Source: CAD feature listing. Evaluate the final solid. Frame: model axes, mm. Give positions to 0.01 mm unless a question says otherwise; leave off trailing zeros. Loops run counter-clockwise (first coordinate to the right, second up) from the corner with the lowest first, then second, coordinate; pieces in that order, holes last. Notation, with made-up numbers: M -34,11 L 10,11 A19 ccw 10,21 Z; hole C -16.5,56 d9. An arc over 180 degrees is marked long. Write item = value, one per line.
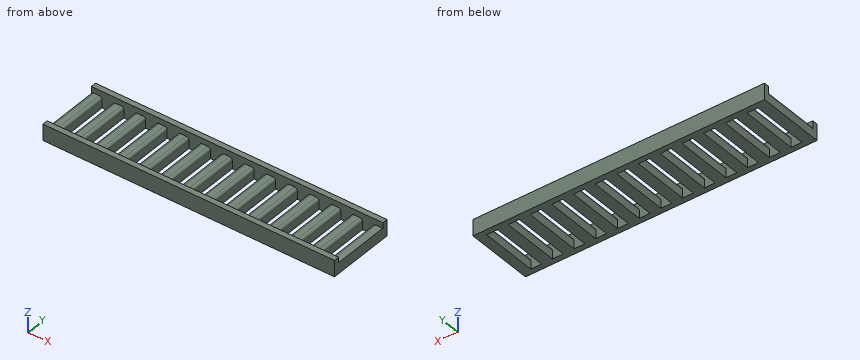
from build123d import *

# Parameters (mm, degrees)
F0_W     = 107.5
F0_H     = 25
F0_W_2   = 4
F0_H_2   = 21
F1_DEPTH = 4
F2_R     = 1
F3_W     = 107.5
F3_H     = 2
F4_DEPTH = 2
F5_R     = 1


# Not quite as in the source:
# - a feature names something its author has since deleted; it is built from what else it names


with BuildPart() as f1:
    # F0 (on Top) → F1 (new body)
    with BuildSketch(Plane.XY):
        with Locations((53.75, 12.5)):
            Rectangle(F0_W, F0_H)
        with Locations((6, 12.5)):
            Rectangle(F0_W_2, F0_H_2, mode=Mode.SUBTRACT)
        with Locations((14, 12.5)):
            Rectangle(F0_W_2, F0_H_2, mode=Mode.SUBTRACT)
        with Locations((22, 12.5)):
            Rectangle(F0_W_2, F0_H_2, mode=Mode.SUBTRACT)
        with Locations((30, 12.5)):
            Rectangle(F0_W_2, F0_H_2, mode=Mode.SUBTRACT)
        with Locations((38, 12.5)):
            Rectangle(F0_W_2, F0_H_2, mode=Mode.SUBTRACT)
        with Locations((46, 12.5)):
            Rectangle(F0_W_2, F0_H_2, mode=Mode.SUBTRACT)
        with Locations((54, 12.5)):
            Rectangle(F0_W_2, F0_H_2, mode=Mode.SUBTRACT)
        with Locations((62, 12.5)):
            Rectangle(F0_W_2, F0_H_2, mode=Mode.SUBTRACT)
        with Locations((70, 12.5)):
            Rectangle(F0_W_2, F0_H_2, mode=Mode.SUBTRACT)
        with Locations((78, 12.5)):
            Rectangle(F0_W_2, F0_H_2, mode=Mode.SUBTRACT)
        with Locations((86, 12.5)):
            Rectangle(F0_W_2, F0_H_2, mode=Mode.SUBTRACT)
        with Locations((94, 12.5)):
            Rectangle(F0_W_2, F0_H_2, mode=Mode.SUBTRACT)
        with Locations((102, 12.5)):
            Rectangle(F0_W_2, F0_H_2, mode=Mode.SUBTRACT)
    extrude(amount=F1_DEPTH)

    # F2
    f2_edges = [f1.edges().sort_by_distance(p)[0] for p in [
        (8, 12.5, 4),
        (12, 12.5, 4),
        (16, 12.5, 4),
        (20, 12.5, 4),
        (24, 12.5, 4),
        (28, 12.5, 4),
        (32, 12.5, 4),
        (36, 12.5, 4),
        (40, 12.5, 4),
        (44, 12.5, 4),
        (48, 12.5, 4),
        (52, 12.5, 4),
        (56, 12.5, 4),
        (60, 12.5, 4),
        (64, 12.5, 4),
        (68, 12.5, 4),
        (72, 12.5, 4),
        (76, 12.5, 4),
        (80, 12.5, 4),
        (84, 12.5, 4),
        (88, 12.5, 4),
        (92, 12.5, 4),
        (96, 12.5, 4),
        (100, 12.5, 4),
        (104, 12.5, 4),
    ]]
    fillet(f2_edges, radius=F2_R)

    # F3 (on face) → F4 (join)
    with BuildSketch(Plane.XY.offset(4)):
        with Locations((53.75, 1)):
            Rectangle(F3_W, F3_H)
        with Locations((53.75, 24)):
            Rectangle(F3_W, F3_H)
    extrude(amount=F4_DEPTH)

    # F5
    f5_edges = [f1.edges().sort_by_distance(p)[0] for p in [
        (4, 12.5, 4),
        (0, 12.5, 4),
    ]]
    fillet(f5_edges, radius=F5_R)


solid = f1.part
1. Cut plane B-B, the plane z = 5. Return the cut outline in (x, y), then the cut area to 3 significant figures.
Derived:
outline = M 0,0 L 107.5,0 L 107.5,2 L 0,2 Z; M 0,23 L 107.5,23 L 107.5,25 L 0,25 Z
area = 430 mm²
2. Cut plane C-C, the plane y = 16.75. Count the separate pieces of the cut face and the enclosed holes in it, then the cut area to 3 significant figures.
Derived:
separate_pieces = 14
enclosed_holes = 0
area = 216 mm²
3. Material intervals for probe 1 along Y at (x, z) = (53, 2.15); probe 2 along Z at (x, y) = (66, 14); probe 3 along Z at (x, y) = (16.5, 10.5), sorted ascending. Write a range as from..to.
Derived:
probe_1 = 0..2, 23..25
probe_2 = 0..4
probe_3 = 0..3.87
4. Cut plane A-A, the plane x = 30. Return the cut outline in (y, z), then the cut area to 3 significant figures.
Derived:
outline = M 0,0 L 2,0 L 2,6 L 0,6 Z; M 23,0 L 25,0 L 25,6 L 23,6 Z
area = 24.0 mm²
5. First-contact query: pin 1 Ø1 at (x, y) = (18, 16.5) entering from +Z; pin 2 Ø1.5 at (x, y) = (92.5, 10.5) entering from +Z. Flat tips, straight axial feed; report the tip coordinate or a pass-through.
Derived:
pin_1 = 4
pin_2 = 3.66
